```python
from build123d import *

# Parameters (mm, degrees)
F1_DEPTH = 38
F3_DEPTH = 25
F4_DEPTH = 7


with BuildPart() as f1:
    # F0 (on Right) → F1 (new body)
    with BuildSketch(Plane.YZ):
        Polygon((15, 19), (15, 20), (15, 24), (11, 24), (11, 15), (11, 6), (15, 6), (15, 10), (15, 11), (21.5, 11), (21.5, 8), (23.5, 8), (23.5, 15), (23.5, 22), (21.5, 22), (21.5, 19), align=None)
    extrude(amount=F1_DEPTH)

    # F2 (on face) → F3 (cut)
    with BuildSketch(Plane(origin=(0, 23.5, 0), x_dir=(-1, 0, 0), z_dir=(0, 1, 0))):
        with BuildLine():
            ThreePointArc((-17.35, 15), (-17.833273811, 16.166726189), (-19, 16.65))
            Line((-19, 16.65), (-19, 13.35))
            ThreePointArc((-19, 13.35), (-17.833273811, 13.833273811), (-17.35, 15))
        make_face()
        with BuildLine():
            Line((-19, 13.35), (-19, 16.65))
            ThreePointArc((-19, 16.65), (-20.65, 15), (-19, 13.35))
        make_face()
    extrude(amount=-F3_DEPTH, mode=Mode.SUBTRACT)

    # F4 (cut): a face of the model
    f4_faces = [f1.faces().sort_by_distance(p)[0] for p in [
        (38, 16.5460526316, 15),
    ]]
    extrude(f4_faces, amount=-F4_DEPTH, mode=Mode.SUBTRACT)


solid = f1.part
```
For this review, take the finished solid that the model builds, in its own axes (mm). A direction names the side the tool comes from. Round coordinates to 2 decimals unless told otherwise and drop trailing zeros. Write each loop counter-clockwise with the first axis right and the second up, starting at its lowest first coordinate (ties: lowest second). Pieces come first, ordered by that corner, then holes. Notation, with made-up numbers: (51, 80.5) - (77, 80.5) arc R22 ccw to (77, 108.5) - close; hole circle Ø3 at (43.5, -14.5). An arc over 180 degrees is marked (long way). Put each result on its own line as item: value.
Q1. Mouldability with a two-part tool opening along Y and no side actions: class faces 1 (the face through (15, 11, 15)), 2 (the face through (15, 15, 21)), 3 (the face through (15, 23, 22)) as released by +Y, released by -Y, zero draft, split by the parting line, or undercut.
Solved:
face 1: released by -Y
face 2: undercut
face 3: zero draft
Q2. We need section B-B (y = 19.75). Give the boundary of the cut face in (x, z).
Solved:
outline: (0, 11) - (31, 11) - (31, 19) - (0, 19) - close; hole circle Ø3.3 at (19, 15)
Q3. Insertion check: pin 1 Ø1.5 at (x, z) = (14.5, 22.5) entering from +Y; pin 2 Ø1.5 at (y, z) = (19.5, 9) entering from -X; pin 3 Ø0.6 at (x, y) = (13, 22) entering from -Z; pin 4 Ø0.6 at (x, y) = (11.5, 22.5) entering from +Z. Each pin has a flat end and moves straight along its axis. Give the tip position at first contact, or say it passes through.
Solved:
pin 1: stops at y = 23.5
pin 2: passes through
pin 3: stops at z = 8
pin 4: stops at z = 22
Q4. We need section D-D (y = 13). Give the boundary of the cut face in (x, z), and give its area (3 significant figures).
Solved:
outline: (0, 6) - (31, 6) - (31, 24) - (0, 24) - close; hole circle Ø3.3 at (19, 15)
area: 549 mm2
Q5. Wall thickness on probe 1 along X at (y, z) = (16.5, 15); probe 2 along Y at (x, z) = (7.5, 23); probe 3 along Y at (x, z) = (17, 21.5): over which ranges is each line inside the solid? List them lowest first.
Solved:
probe 1: x = 0 to 17.35, 20.65 to 31
probe 2: y = 11 to 15
probe 3: y = 11 to 15, 21.5 to 23.5
Q6. Machinability: for faces 4 (the face through (15, 18, 19)), 5 (the face through (15, 21.5, 10)), 6 (the face through (15, 22, 8)), 7 (the face through (0, 16, 15)), 8 (the face through (15, 13, 24)), which of the approach directions +Z, -Z, +X, -X, +Y, -Y give a long, thin tool a straight path to every point of the face, cutting with its end or side? Answer none if there is none.
Solved:
face 4: +Z, +X, -X
face 5: -Z, +X, -X
face 6: -Z, +X, -X, +Y
face 7: +Z, -Z, -X, +Y, -Y
face 8: +Z, +X, -X, +Y, -Y
Q7. We need section A-A (z = 9.5). Give the boundary of the cut face in (x, y), and give its area (3 significant figures).
Solved:
outline: (0, 11) - (31, 11) - (31, 15) - (0, 15) - close; (0, 21.5) - (31, 21.5) - (31, 23.5) - (0, 23.5) - close
area: 186 mm2
Q8. We need section C-C (x = 25). Give the boundary of the cut face in (y, z).
Solved:
outline: (11, 6) - (15, 6) - (15, 11) - (21.5, 11) - (21.5, 8) - (23.5, 8) - (23.5, 22) - (21.5, 22) - (21.5, 19) - (15, 19) - (15, 24) - (11, 24) - close
